Geometry: final body of the model. Coordinates: model frame, mm. Coordinates: 2 decimals unless noted, no trailing zeros. Order: outer loops, then holes, each group sorted by start corner. A loop starts at its lowest first (then second) coordinate and runs counter-clockwise, first axis right, second up. Notation, with made-up numbers: (-5.75, -21.5) -> (12.25, -21.5) arc R28 cw to (12.25, 12.5) -> close; hole circle Ø11 at (88, 49). An arc over 180 degrees is marked (long way). Answer in a Markdown table with one row per item. Add a question column.
1) Section query A-A on y = 80. Return the cut outline in (x, z), then the cut area to 4 significant figures.
2) Ray query, line 1 (Y direction, x = -49.5, z = 2.65); line 2 (Y direction, x = -44.5, z = 0.3); line 3 (Y direction, x = -36, z = 1.45). Return the intervals inside material, ascending. Write a range as from..to.
3) Section query C-C on z = 2.2. Return the cut outline in (x, y), then the cut area to 3 significant figures.
4) Section query D-D on y = 146. Return the cut outline in (x, z).
5) Contact query for a flat-ended pin moving along its axis: P1, Ø0.9, axis at x = -36, z = 1, coming from the +Y side. Output: stop coordinate, or through.
6) Section query B-B on x = -33. Return the cut outline in (y, z), then the cut area to 3 significant figures.
Autodesk Inventor part; units mm, degrees
ref_plane "YZ Plane" through (0, 0, 0) normal (1, 0, 0) x (0, 1, 0)
ref_plane "XZ Plane" through (0, 0, 0) normal (0, 1, 0) x (-1, 0, 0)
ref_plane "XY Plane" through (0, 0, 0) normal (0, 0, 1) x (1, 0, 0)
sketch "Sketch1" plane through (0, 0, 0) normal (0, 0, 1) x (1, 0, 0)
  circle A0 centre (1008.2886, -225.2) radius 1095
  line L0 (-27.5, 131.7988) -> (-27.5, 31.7988)
  line L1 (-43.3188, 130) -> (-43.3188, 30)
  line L2 (-56.5579, 30) -> (-56.5579, 130)
  line L3 (-27.5, 130) -> (-56.5579, 130)
  line L4 (-27.5, 80) -> (-56.5579, 80)
  line L5 (-27.5, 30) -> (-56.5579, 30)
  line L6 (-111.5579, 160) -> (0, 160)
  line L7 (0, 160) -> (0, 0)
  line L8 (0, 0) -> (-111.5579, 0)
  line L9 (-111.5579, 0) -> (-111.5579, 160)
  point P0 (0, 0)
  point P1 (-43.3188, 80)
  dimension "d4" = 2190
  dimension "d10" = 50
  dimension "d11" = 50
  dimension "d21" = 305.2
  dimension "d36" = 30
  dimension "d37" = 30
  dimension "d38" = 27.5
  dimension "d39" = 55
extrude "Extrusion1" add sketch "Sketch1" along normal blind 3 contours L6 L7 L8 A0 L5 L1 L4 L0 | A0 L3 L2 L8 L9 L6 | L0 L4 A0 | A0 L1 L3 | L2 L4 A0 | A0 L1 L5 | L4 L2 L3 L1
hole "Hole1" at (-27.5, 130, 0) at (-43.3188, 80, 0) at (-56.5579, 30, 0) at (-43.3188, 130, 0) at (-27.5, 80, 0) at (-43.3188, 30, 0) at (-56.5579, 80, 0) direction (0, 0, 1) diameter 12 end through all
sketch "Sketch2" plane through (0, 0, 0) normal (0, 0, -1) x (-1, 0, 0)
  circle A0 centre (27.5, 130) radius 6
  circle A1 centre (43.3188, 130) radius 6
  line L0 (27.5, 124) -> (43.3188, 124)
  circle A2 centre (27.5, 130) radius 6
  line L1 (27.5, 136) -> (43.3188, 136)
  line L2 (27.5, 136) -> (27.5, 124)
  line L3 (43.3188, 124) -> (43.3188, 136)
  line L4 (27.5, 86) -> (56.5579, 86)
  line L5 (27.5, 74) -> (56.5579, 74)
  circle A3 centre (27.5, 80) radius 6
  circle A4 centre (56.5579, 80) radius 6
  line L6 (27.5, 86) -> (27.5, 74)
  line L7 (56.5579, 74) -> (56.5579, 86)
  line L8 (43.3188, 36) -> (56.5579, 36)
  line L9 (43.3188, 24) -> (56.5579, 24)
  circle A5 centre (43.3188, 30) radius 6
  circle A6 centre (56.5579, 30) radius 6
  line L10 (43.3188, 24) -> (43.3188, 36)
  line L11 (56.5579, 24) -> (56.5579, 36)
  point P0 (0, 0)
extrude "Extrusion2" cut sketch "Sketch2" against normal blind 3 contours A0 L1 A1 L0 | L4 A4 L5 A3 | L8 A6 L9 A5
sketch "Sketch3" plane through (0, 0, 3) normal (0, 0, 1) x (1, 0, 0)
  line L0 (-111.5579, 160) -> (-111.5579, 0)
  line L1 (0, 160) -> (-111.5579, 160)
  line L2 (-111.5579, 0) -> (0, 0)
  line L3 (-56.5579, 86) -> (-27.5, 86)
  line L4 (-27.5, 124) -> (-43.3188, 124)
  line L5 (-27.5, 74) -> (-56.5579, 74)
  line L6 (-56.5579, 36) -> (-43.3188, 36)
  point P0 (-91.5579, 146)
  point P1 (-91.5579, 14)
  dimension "d51" = 20
  dimension "d52" = 14
  dimension "d53" = 14
  dimension "d54" = 20
hole "Hole2" at (-91.5579, 14, 3) at (-91.5579, 146, 3) direction (0, 0, -1) diameter 8 end through all
fillet "Fillet2" radius 40 2 edges at (0, 0, 1.5) (0, 160, 1.5)
fillet "Fillet3" radius 8 2 edges at (-111.5579, 0, 1.5) (-111.5579, 160, 1.5)
equation "\"d11\" = d10"
properties part number "adjust_sheet" material "Steel, Mild"
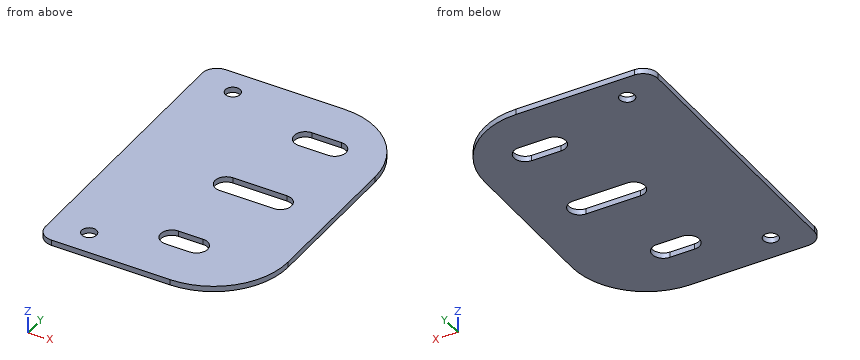
Result:
| question | item | result |
|---|---|---|
| 1 | outline | (-111.56, 0) -> (-62.56, 0) -> (-62.56, 3) -> (-111.56, 3) -> close; (-21.5, 0) -> (0, 0) -> (0, 3) -> (-21.5, 3) -> close |
| 1 | area | 211.5 mm2 |
| 2 | line 1 | 0..24, 36..74, 86..160 |
| 2 | line 2 | 0..24, 36..74, 86..124.12, 135.88..160 |
| 2 | line 3 | 0.2..74, 86..124, 136..159.8 |
| 3 | outline | (-111.56, 8) arc R8 ccw to (-103.56, 0) -> (-40, 0) arc R40 ccw to (0, 40) -> (0, 120) arc R40 ccw to (-40, 160) -> (-103.56, 160) arc R8 ccw to (-111.56, 152) -> close; hole circle Ø8 at (-91.56, 14); hole circle Ø8 at (-91.56, 146); hole (-56.56, 24) -> (-43.32, 24) arc R6 ccw to (-43.32, 36) -> (-56.56, 36) arc R6 ccw to start; hole (-56.56, 74) -> (-27.5, 74) arc R6 ccw to (-27.5, 86) -> (-56.56, 86) arc R6 ccw to start; hole (-43.32, 124) -> (-27.5, 124) arc R6 ccw to (-27.5, 136) -> (-43.32, 136) arc R6 ccw to start |
| 3 | area | 16,000 mm2 |
| 4 | outline | (-111.56, 0) -> (-95.56, 0) -> (-95.56, 3) -> (-111.56, 3) -> close; (-87.56, 0) -> (-9.6, 0) -> (-9.6, 3) -> (-87.56, 3) -> close |
| 5 | P1 | y = 159.84 |
| 6 | outline | (0.62, 0) -> (74, 0) -> (74, 3) -> (0.62, 3) -> close; (86, 0) -> (124, 0) -> (124, 3) -> (86, 3) -> close; (136, 0) -> (159.38, 0) -> (159.38, 3) -> (136, 3) -> close |
| 6 | area | 404 mm2 |
